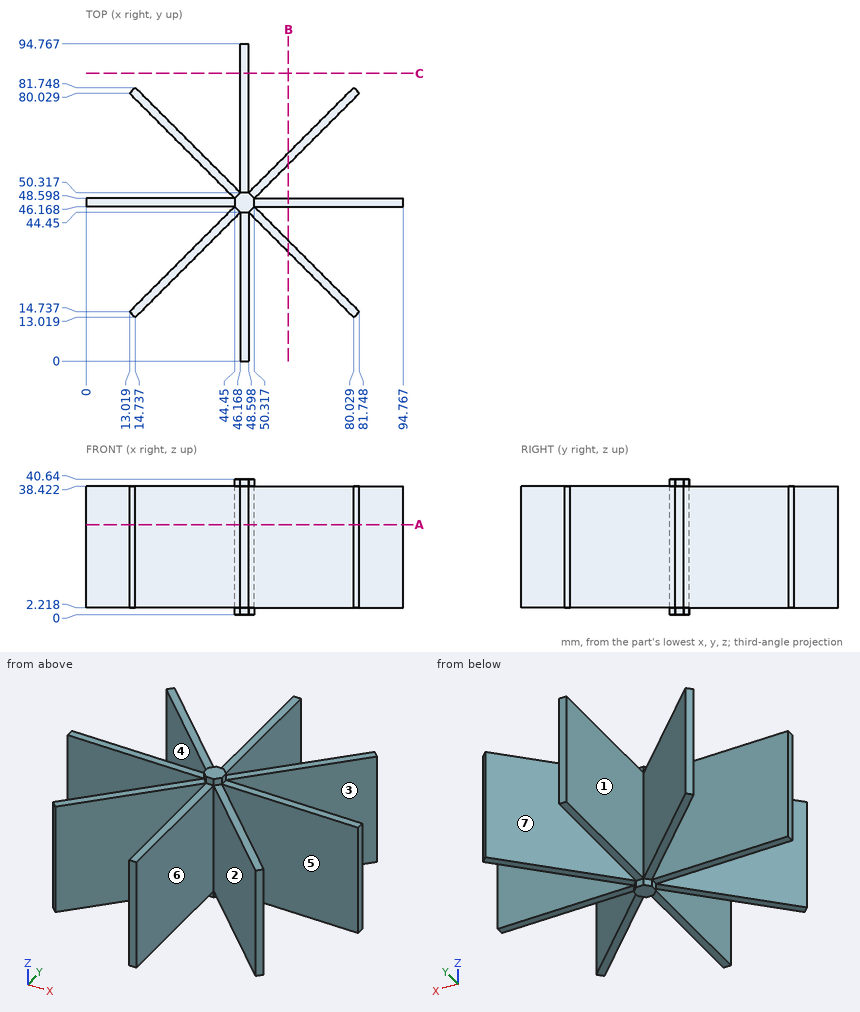
The drawing under review shows one solid part. Ordinate dimensions are in mm from its lowest x, y, z. A direction names the side the tool comes from. Round coordinates to 2 decimals unless told otherwise and drop trailing zeros. Loops run counter-clockwise (first coordinate to the right, second up) from the corner with the lowest first, then second, coordinate; pieces in that order, holes last. Notation, with made-up numbers: (46, 20.25) - (87, 20.25) arc R16 cw to (87, 28.25) - close; hole circle Ø11 at (57, 22.25). An arc over 180 degrees is marked (long way). One line per question, with ' | ' between items.
Q1. Take a section at B-B (x = 60.5). Give the boundary of the cut face in (y, z) (1 decimal), and give its area (3 significant figures).
Taken from the geometry:
outline: (32.5, 2.2) - (36, 2.2) - (36, 38.4) - (32.5, 38.4) - close; (46.2, 2.2) - (48.6, 2.2) - (48.6, 38.4) - (46.2, 38.4) - close; (58.8, 2.2) - (62.2, 2.2) - (62.2, 38.4) - (58.8, 38.4) - close | area: 337 mm²
Q2. The part is to be moulded in two halves that separate along Y. For the marked faces 5, 6 and 7, say which applies: released by +Y, released by -Y, zero draft, split by the parting line, or undercut.
Taken from the geometry:
face 5: undercut | face 6: zero draft | face 7: released by +Y
Q3. For line 1 along X through (y, z) = (81, 33) (1 decimal); line 2 along X through (y, z) = (84, 8.5); line 3 along Z through (x, y) = (57.5, 48.5), list the stretches that pass through material, from the lowest coordinate up. Write a range as [from, to].
Taken from the geometry:
line 1: x = [14, 15.5], [46.2, 48.6], [79.3, 80.8] | line 2: x = [46.17, 48.6] | line 3: z = [2.22, 38.42]
Q4. Tool access review of the marked faces 1, 2, 3 and 4: name each direction out of +Z, -Z, +X, -X, +Y, -Y from which nothing blocks a thin tool from reaching the whole face with its end or side.
Taken from the geometry:
face 1: +Z, -Z, +Y | face 2: +Z, -Z, -Y | face 3: +Z, -Z, +X | face 4: +Z, -Z, -X
Q5. Take a section at C-C (y = 86). Give the boundary of the cut face in (x, z).
Taken from the geometry:
outline: (46.17, 2.22) - (48.6, 2.22) - (48.6, 38.42) - (46.17, 38.42) - close
Q6. Take a section at A-A (z = 27). Give the boundary of the cut face in (x, y).
Taken from the geometry:
outline: (0, 46.17) - (44.45, 46.17) - (13.02, 14.74) - (14.74, 13.02) - (46.17, 44.45) - (46.17, 0) - (48.6, 0) - (48.6, 44.45) - (80.03, 13.02) - (81.75, 14.74) - (50.32, 46.17) - (94.77, 46.17) - (94.77, 48.6) - (50.32, 48.6) - (81.75, 80.03) - (80.03, 81.75) - (48.6, 50.32) - (48.6, 94.77) - (46.17, 94.77) - (46.17, 50.32) - (14.74, 81.75) - (13.02, 80.03) - (44.45, 48.6) - (0, 48.6) - close
Q7. For pin 1 (6 mm diameter, centred on y = 58.5, z = 24, fed in from -X); pin 2 (12 mm diameter, centred on x = 83.5, y = 21, fed in from +Z); pin 3 (12 mm diameter, centred on x = 18.5, y = 48.5, fed in from -Z); pin 4 (6 mm diameter, centred on x = 70.5, y = 61.5, fed in from +Z), all flat-tipped, find the tip position at first contact; note any pin that passes through.
Taken from the geometry:
pin 1: stops at x = 31.55 | pin 2: stops at z = 38.42 | pin 3: stops at z = 2.22 | pin 4: passes through
